from build123d import *

# Parameters (mm, degrees)
SKETCH1_W               = 10
SKETCH1_H               = 15
BOSS_EXTRUDE1_DEPTH     = 15
CUT_EXTRUDE1_DEPTH      = 18.5
CUT_EXTRUDE1_DEPTH_BACK = 18.5
SKETCH2_W               = 0.7
SKETCH2_H               = 10
SKETCH3_W               = 5
SKETCH3_H               = 2.3
SKETCH3_W_2             = 10
SKETCH3_H_2             = 2.5
BOSS_EXTRUDE2_DEPTH     = 15
CUT_EXTRUDE2_DEPTH      = 24.452078799
CUT_EXTRUDE2_DEPTH_BACK = 24.452078799
SKETCH4_W               = 1.5
SKETCH4_H               = 2.5
CUT_EXTRUDE3_DEPTH      = 21.615528128
CUT_EXTRUDE3_DEPTH_BACK = 21.615528128
SKETCH5_W               = 0.7
SKETCH5_H               = 2.5


with BuildPart() as part:
    # Sketch1 → Boss-Extrude1 (new body)
    with BuildSketch(Plane.XY):
        Rectangle(SKETCH1_W, SKETCH1_H)
    extrude(amount=BOSS_EXTRUDE1_DEPTH)

    # Sketch2 → Cut-Extrude1 (cut, two sides: drawn at the far end of the back side and taken through both)
    with BuildSketch(Plane.XY.offset(15).offset(-CUT_EXTRUDE1_DEPTH_BACK)):
        with Locations((0, -2.5)):
            Rectangle(SKETCH2_W, SKETCH2_H)
    extrude(amount=CUT_EXTRUDE1_DEPTH + CUT_EXTRUDE1_DEPTH_BACK, mode=Mode.SUBTRACT)

    # Sketch3 → Boss-Extrude2 (add)
    with BuildSketch(Plane.XY.offset(15)):
        with Locations((-7.5, -3.85)):
            Rectangle(SKETCH3_W, SKETCH3_H)
        with Locations((7.5, -3.85)):
            Rectangle(SKETCH3_W, SKETCH3_H)
        with Locations((0, 8.75)):
            Rectangle(SKETCH3_W_2, SKETCH3_H_2)
    extrude(amount=-BOSS_EXTRUDE2_DEPTH)

    # Sketch4 → Cut-Extrude2 (cut, two sides: drawn at the far end of the back side and taken through both)
    with BuildSketch(Plane.ZY.offset(5).offset(-CUT_EXTRUDE2_DEPTH_BACK)):
        with Locations((0.75, -6.25)):
            Rectangle(SKETCH4_W, SKETCH4_H)
        with Locations((14.25, -6.25)):
            Rectangle(SKETCH4_W, SKETCH4_H)
    extrude(amount=CUT_EXTRUDE2_DEPTH + CUT_EXTRUDE2_DEPTH_BACK, mode=Mode.SUBTRACT)

    # Sketch5 → Cut-Extrude3 (cut, two sides: drawn at the far end of the back side and taken through both)
    with BuildSketch(Plane(origin=(0, 0, 0), x_dir=(-1, 0, 0), z_dir=(0, 0, -1)).offset(-CUT_EXTRUDE3_DEPTH_BACK)):
        with Locations((4.65, -6.25)):
            Rectangle(SKETCH5_W, SKETCH5_H)
        with Locations((-4.65, -6.25)):
            Rectangle(SKETCH5_W, SKETCH5_H)
    extrude(amount=CUT_EXTRUDE3_DEPTH + CUT_EXTRUDE3_DEPTH_BACK, mode=Mode.SUBTRACT)


solid = part.part
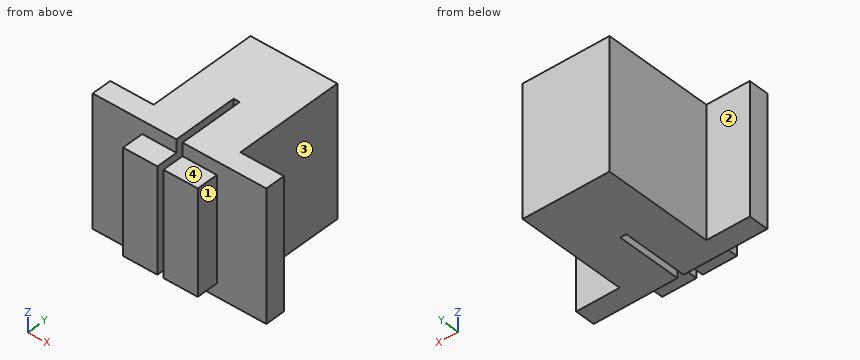
Model file for the job. Use its own axes, mm. Face numbers are marked on the shaded views. A direction names the side the tool comes from. Give positions to 0.01 mm unless a question says otherwise; leave off trailing zeros. Loops run counter-clockwise (first coordinate to the right, second up) from the corner with the lowest first, then second, coordinate; pieces in that order, holes last. Notation, with made-up numbers: (22, -13) - (49, -13) arc R16 ccw to (49, 12) - close; hole circle Ø11 at (54.25, 88). An arc over 180 degrees is marked (long way). Use one line per item in the form item = value.
(1) 3-axis set-ups, long thin cutter, end or side, ignore diameter. For the marked faces 1, 2, 3 and 4: which of +Z, -Z, +X, -X, +Y, -Y reach the whole face in a straight line?
Determined:
face_1 = +Z, -Z, +X, -Y
face_2 = +Z, -Z, -X, +Y
face_3 = +Z, -Z, +X, +Y
face_4 = +Z, +X, -X, -Y
(2) Cut at C-C (x = -2.75). Give the cut face in (y, z), then the cut area to 3 significant figures.
Determined:
outline = (-7.5, 1.5) - (-5, 1.5) - (-5, 0) - (10, 0) - (10, 15) - (-5, 15) - (-5, 13.5) - (-7.5, 13.5) - close
area = 255 mm^2
(3) Cut at D-D (y = -3.5). Give the cut face in (x, z).
Determined:
outline = (-10, 0) - (-0.35, 0) - (-0.35, 15) - (-10, 15) - close; (0.35, 0) - (10, 0) - (10, 15) - (0.35, 15) - close
(4) Drill centre lines: L1, parallel to X at y = -1.5, z = 2; L2, parallel to X at y = -6.5, z = 6.25; L3, parallel to Y at x = -9, z = 7. Where is each one in solid material? Low to high.
Determined:
L1 = -5 to -0.35, 0.35 to 5
L2 = -4.3 to -0.35, 0.35 to 4.3
L3 = -5 to -2.7
(5) Drop flat-ended pins along their axis: P1, Ø6, axis at x = 7.5, z = 9, coming from the -Y side; P2, Ø2, axis at y = 2, z = 3.5, coming from the +X side; P3, Ø1.2, axis at x = -3, y = -6, coming from the -Z side. Give the stop position or say it passes through.
Determined:
P1 = -5
P2 = 5
P3 = 1.5
(6) Cut at B-B (z = 1). Give the cut face in (x, y).
Determined:
outline = (-10, -5) - (-0.35, -5) - (-0.35, 2.5) - (0.35, 2.5) - (0.35, -5) - (10, -5) - (10, -2.7) - (5, -2.7) - (5, 10) - (-5, 10) - (-5, -2.7) - (-10, -2.7) - close
(7) Cut at A-A (y = -6). Give the cut face in (x, z).
Determined:
outline = (-4.3, 1.5) - (-0.35, 1.5) - (-0.35, 13.5) - (-4.3, 13.5) - close; (0.35, 1.5) - (4.3, 1.5) - (4.3, 13.5) - (0.35, 13.5) - close
